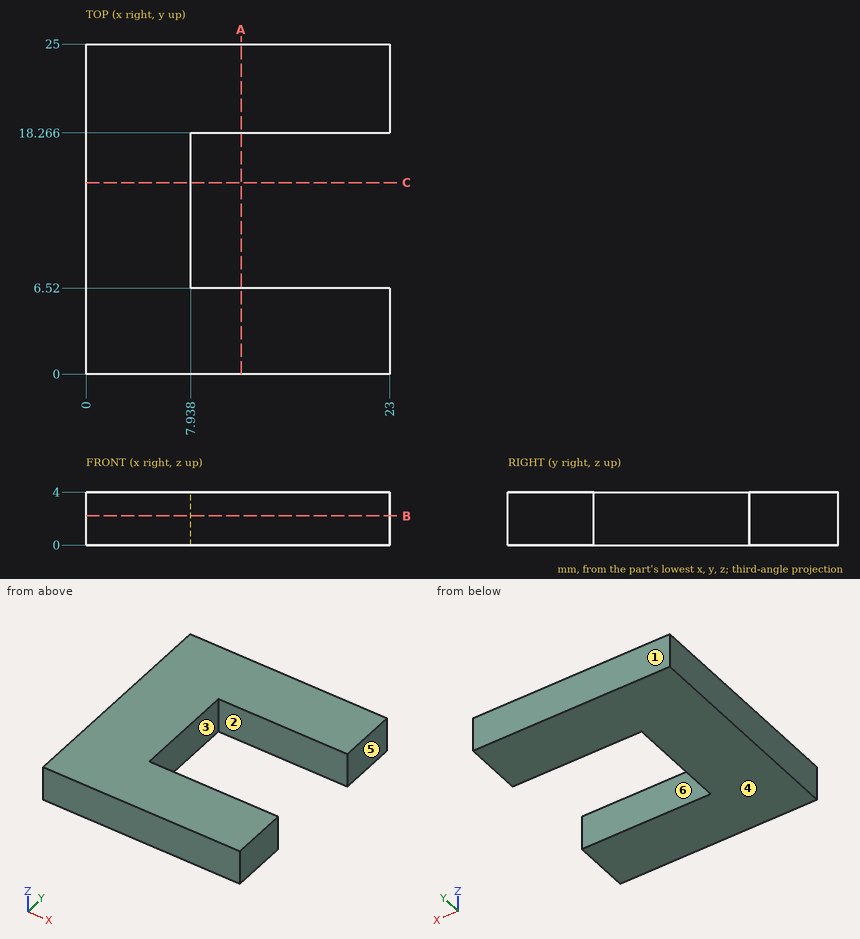
Study the drawing (mm; zero at the part's minimum x, y, z) and answer. A direction names the side the tool comes from. Give positions to 0.01 mm unless a question says otherwise; leave off trailing zeros. Write each loop counter-clockwise with the first axis right and the second up, starting at its lowest first coordinate (ties: lowest second). Pieces come first, ordered by that corner, then holes. Notation, with made-up numbers: (82, 17) - (108, 17) arc R18 ccw to (108, 41) - close; hole circle Ø5 at (1.5, -18). An arc over 180 degrees is marked (long way). Use CSV: the item, a comma, the result in double quotes. Start each with the question number.
(1) Consider line 1 along Y through (x, z) = (14.75, 1.95) (1 decimal); line 2 along X through (y, z) = (8.5, 3.7). Determine where each line is inside the solid, lowest interval first.
(2) Find section B-B (z = 2.2). Give the vertices of the cut face in (x, y) (1 decimal).
(3) Find section A-A (x = 11.75). Give the vertices of the cut face in (y, z) (1 decimal).
(4) Find section C-C (y = 14.5). Give the vertices of the cut face in (x, z).
(5) Determine the mould class of the marked faces 1, 2, 3 and 4 for opening direction Y: +Y half, -Y half, draft (parallel to the pull), parting line (faces both ways), or undercut.
(6) For the marked faces 5 and 6, determine the directions among +Z, -Z, +X, -X, +Y, -Y from which every point of the face is accessible in a straight line to the end or side of a thin tool.
(7) Given P1, Ø1.5, axis at y = 12.5, z = 0.5, coming from the +X side, flat-ended and moving along its own axis, determine where the tip first touches the part or whether it passes through.
Findings below:
1,line 1,"0 to 6.5, 18.3 to 25"
1,line 2,"0 to 7.94"
2,outline,"(0, 0) - (23, 0) - (23, 6.5) - (7.9, 6.5) - (7.9, 18.3) - (23, 18.3) - (23, 25) - (0, 25) - close"
3,outline,"(0, 0) - (6.5, 0) - (6.5, 4) - (0, 4) - close; (18.3, 0) - (25, 0) - (25, 4) - (18.3, 4) - close"
4,outline,"(0, 0) - (7.94, 0) - (7.94, 4) - (0, 4) - close"
5,face 1,"+Y half"
5,face 2,"undercut"
5,face 3,"undercut"
5,face 4,"draft"
6,face 5,"+Z, -Z, +X, +Y, -Y"
6,face 6,"+Z, -Z, +X"
7,P1,"x = 7.94"
